from build123d import *

# Parameters (mm, degrees)
BOSS_EXTRUDE1_DEPTH            = 4.8
BOSS_EXTRUDE3_DEPTH            = 4.8
M3_CLEARANCE_HOLE2_D           = 3.4
M3_CLEARANCE_HOLE2_CSINK_D     = 3.45
M3_CLEARANCE_HOLE2_CSINK_ANGLE = 90
BOSS_EXTRUDE4_DEPTH            = 4.8
SKETCH11_W                     = 23
SKETCH11_H                     = 12.75
CUT_EXTRUDE1_DEPTH             = 4.8
M2_CLEARANCE_HOLE1_D           = 2.4
M2_CLEARANCE_HOLE1_CSINK_D     = 2.45
M2_CLEARANCE_HOLE1_CSINK_ANGLE = 90
CUT_EXTRUDE2_DEPTH             = 4.8
SKETCH16_W                     = 4.8
SKETCH16_H                     = 7
BOSS_EXTRUDE6_DEPTH            = 11
SKETCH17_R                     = 1.225
CUT_EXTRUDE3_DEPTH             = 11
CUT_EXTRUDE4_DEPTH             = 1.75


with BuildPart() as part:
    # Sketch1 → Boss-Extrude1 (new body)
    with BuildSketch(Plane(origin=(0, 0, 0), x_dir=(1, 0, 0), z_dir=(0, 1, 0))):
        with BuildLine():
            Line((6.83, 0), (-6.83, 0))
            ThreePointArc((-6.83, 0), (-8.951320344, -0.878679656), (-9.83, -3))
            Line((-9.83, -3), (-9.83, -7.63))
            ThreePointArc((-9.83, -7.63), (-10.708679656, -9.751320344), (-12.83, -10.63))
            Line((-12.83, -10.63), (-12.83, -16.63))
            Line((-12.83, -16.63), (12.83, -16.63))
            Line((12.83, -16.63), (12.83, -10.63))
            ThreePointArc((12.83, -10.63), (10.708679656, -9.751320344), (9.83, -7.63))
            Line((9.83, -7.63), (9.83, -3))
            ThreePointArc((9.83, -3), (8.951320344, -0.878679656), (6.83, 0))
        make_face()
    extrude(amount=BOSS_EXTRUDE1_DEPTH)

    # Sketch9 → Boss-Extrude3 (add)
    with BuildSketch(Plane(origin=(0, 4.8, 0), x_dir=(1, 0, 0), z_dir=(0, 1, 0))):
        with BuildLine():
            Line((12.83, -16.63), (12.83, -10.63))
            Line((12.83, -10.63), (20.51, -10.63))
            ThreePointArc((20.51, -10.63), (22.631320344, -9.751320344), (23.51, -7.63))
            Line((23.51, -7.63), (23.51, -5.44))
            ThreePointArc((23.51, -5.44), (24.388679656, -3.318679656), (26.51, -2.44))
            Line((26.51, -2.44), (27.36, -2.44))
            ThreePointArc((27.36, -2.44), (29.481320344, -1.561320344), (30.36, 0.56))
            Line((30.36, 0.56), (30.36, 6.56))
            Line((30.36, 6.56), (36.36, 6.56))
            Line((36.36, 6.56), (36.36, -16.63))
            Line((36.36, -16.63), (12.83, -16.63))
        make_face()
    extrude(amount=-BOSS_EXTRUDE3_DEPTH)

    # M3 Clearance Hole2 (through all)
    with Locations(Plane(origin=(0, 4.8, 0), x_dir=(1, 0, 0), z_dir=(0, 1, 0))):
        with Locations((0, -4.05), (30.821320344, -9.051320344)):
            CounterSinkHole(M3_CLEARANCE_HOLE2_D / 2, M3_CLEARANCE_HOLE2_CSINK_D / 2, counter_sink_angle=M3_CLEARANCE_HOLE2_CSINK_ANGLE)

    # Sketch10 → Boss-Extrude4 (add)
    with BuildSketch(Plane(origin=(0, 4.8, 0), x_dir=(1, 0, 0), z_dir=(0, 1, 0))):
        Polygon((-12.83, -16.63), (-12.83, -41.63), (77.88, -41.63), (77.88, 6.56), (36.36, 6.56), (36.36, -16.63), align=None)
    extrude(amount=-BOSS_EXTRUDE4_DEPTH)

    # Sketch11 → Cut-Extrude1 (cut)
    with BuildSketch(Plane(origin=(0, 4.8, 0), x_dir=(1, 0, 0), z_dir=(0, 1, 0))):
        with Locations((38.94, -30.255)):
            Rectangle(SKETCH11_W, SKETCH11_H)
    extrude(amount=-CUT_EXTRUDE1_DEPTH, mode=Mode.SUBTRACT)

    # M2 Clearance Hole1 (through all)
    with Locations(Plane(origin=(0, 4.8, 0), x_dir=(1, 0, 0), z_dir=(0, 1, 0))):
        with Locations((25.04, -30.255), (52.84, -30.255)):
            CounterSinkHole(M2_CLEARANCE_HOLE1_D / 2, M2_CLEARANCE_HOLE1_CSINK_D / 2, counter_sink_angle=M2_CLEARANCE_HOLE1_CSINK_ANGLE)

    # Sketch14 → Cut-Extrude2 (cut)
    with BuildSketch(Plane(origin=(0, 4.8, 0), x_dir=(1, 0, 0), z_dir=(0, 1, 0))):
        Polygon((-12.83, -16.59), (8.952290106, -41.63), (-12.83, -41.63), align=None)
        Polygon((36.36, 6.56), (77.88, -41.63), (77.88, 6.56), align=None)
    extrude(amount=-CUT_EXTRUDE2_DEPTH, mode=Mode.SUBTRACT)

    # Chamfer2
    # the kernel refuses this chamfer: 2, 1.418117079 mm, written as the material it takes off along each edge
    with BuildSketch(Plane(origin=(75.517763148, 3.466666667, 40.45827363), x_dir=(-0.07414602746519786, 0, 0.9972473948881141), z_dir=(0.5424620475376688, 0.83911156735298, 0.040332425115101794))) as chamfer2_piece_1:
        Polygon((-0.420862971, 1.22558177), (1.098498339, 1.22558177), (-0.677635367, -2.451163541), align=None)
    extrude(amount=2.692247612, mode=Mode.SUBTRACT)
    with BuildSketch(Plane(origin=(75.517763148, 1.333333333, 40.45827363), x_dir=(-0.07414602746519786, 0, 0.9972473948881141), z_dir=(0.5424620475376688, -0.83911156735298, 0.040332425115102044))) as chamfer2_piece_2:
        Polygon((-0.420862971, -1.22558177), (1.098498339, -1.22558177), (-0.677635367, 2.451163541), align=None)
    extrude(amount=2.692247612, mode=Mode.SUBTRACT)
    with BuildSketch(Plane(origin=(3.80892413, 4.8, 41.63), x_dir=(0, 0.02749587661058651, -0.9996219169112968), z_dir=(1, 0, 0))) as chamfer2_piece_3:
        with BuildLine():
            Line((2.05734639, 0), (-0.11309431, -2.054235587))
            Line((-0.11309431, -2.054235587), (-0.153079186, -2.053135752))
            ThreePointArc((-0.153079186, -2.053135752), (-0.068258454, -1.026795659), (-0.039984877, 0.001099835))
            Line((-0.039984877, 0.001099835), (0.001099835, 0.039984877))
            ThreePointArc((0.001099835, 0.039984877), (1.028995329, 0.011711299), (2.058446225, 0.039984877))
            Line((2.058446225, 0.039984877), (2.05734639, 0))
        make_face()
    extrude(amount=79.214441846, mode=Mode.SUBTRACT)
    with BuildSketch(Plane(origin=(-16.205706468, 4.8, 12.709430531), x_dir=(0.7541952701172161, 0.027495876610586487, -0.6560742879447683), z_dir=(0.6563224323571792, 0, 0.754480526445021))) as chamfer2_piece_4:
        with BuildLine():
            Line((2.05734639, 0), (-0.11309431, -2.054235587))
            Line((-0.11309431, -2.054235587), (-0.153079186, -2.053135752))
            ThreePointArc((-0.153079186, -2.053135752), (-0.068258454, -1.026795659), (-0.039984877, 0.001099835))
            Line((-0.039984877, 0.001099835), (0.001099835, 0.039984877))
            ThreePointArc((0.001099835, 0.039984877), (1.028995329, 0.011711299), (2.058446225, 0.039984877))
            Line((2.058446225, 0.039984877), (2.05734639, 0))
        make_face()
    extrude(amount=43.475129959, mode=Mode.SUBTRACT)
    with BuildSketch(Plane(origin=(-16.205706468, 0, 12.709430531), x_dir=(0.7541952701172161, -0.02749587661058636, -0.6560742879447683), z_dir=(0.6563224323571792, 0, 0.754480526445021))) as chamfer2_piece_5:
        with BuildLine():
            Line((2.05734639, 0), (-0.11309431, 2.054235587))
            Line((-0.11309431, 2.054235587), (-0.153079186, 2.053135752))
            ThreePointArc((-0.153079186, 2.053135752), (-0.068258454, 1.026795659), (-0.039984877, -0.001099835))
            Line((-0.039984877, -0.001099835), (0.001099835, -0.039984877))
            ThreePointArc((0.001099835, -0.039984877), (1.028995329, -0.011711299), (2.058446225, -0.039984877))
            Line((2.058446225, -0.039984877), (2.05734639, 0))
        make_face()
    extrude(amount=43.475129959, mode=Mode.SUBTRACT)
    with BuildSketch(Plane(origin=(33.002764366, 4.8, -10.456560337), x_dir=(-0.7573031224660502, 0.027495876610586473, 0.6524844499852744), z_dir=(0.6527312366273116, 0, 0.757589554264696))) as chamfer2_piece_6:
        with BuildLine():
            Line((2.05734639, 0), (-0.11309431, 2.054235587))
            Line((-0.11309431, 2.054235587), (-0.153079186, 2.053135752))
            ThreePointArc((-0.153079186, 2.053135752), (-0.068258454, 1.026795659), (-0.039984877, -0.001099835))
            Line((-0.039984877, -0.001099835), (0.001099835, -0.039984877))
            ThreePointArc((0.001099835, -0.039984877), (1.028995329, -0.011711299), (2.058446225, -0.039984877))
            Line((2.058446225, -0.039984877), (2.05734639, 0))
        make_face()
    extrude(amount=73.896373517, mode=Mode.SUBTRACT)
    with BuildSketch(Plane(origin=(33.002764366, 0, -10.456560337), x_dir=(-0.7573031224660502, -0.02749587661058634, 0.6524844499852744), z_dir=(0.6527312366273116, 0, 0.757589554264696))) as chamfer2_piece_7:
        with BuildLine():
            Line((2.05734639, 0), (-0.11309431, -2.054235587))
            Line((-0.11309431, -2.054235587), (-0.153079186, -2.053135752))
            ThreePointArc((-0.153079186, -2.053135752), (-0.068258454, -1.026795659), (-0.039984877, 0.001099835))
            Line((-0.039984877, 0.001099835), (0.001099835, 0.039984877))
            ThreePointArc((0.001099835, 0.039984877), (1.028995329, 0.011711299), (2.058446225, 0.039984877))
            Line((2.058446225, 0.039984877), (2.05734639, 0))
        make_face()
    extrude(amount=73.896373517, mode=Mode.SUBTRACT)
    with BuildSketch(Plane(origin=(77.88, 9.943365976, 41.63), x_dir=(-0.6316538610797438, 0, -0.7752505400082296), z_dir=(0, -1, 0))) as chamfer2_piece_8:
        with BuildLine():
            Line((2.05734639, 0), (0.837656572, -1.154387784))
            Line((0.837656572, -1.154387784), (0.80664655, -1.179653939))
            ThreePointArc((0.80664655, -1.179653939), (0.418742927, -0.57726344), (-0.031010022, -0.025266154))
            Line((-0.031010022, -0.025266154), (0.001099835, 0.039984877))
            ThreePointArc((0.001099835, 0.039984877), (1.028995329, 0.011711299), (2.058446225, 0.039984877))
            Line((2.058446225, 0.039984877), (2.05734639, 0))
        make_face()
    extrude(amount=15.086731952, mode=Mode.SUBTRACT)
    with BuildSketch(Plane(origin=(3.80892413, 0, 41.63), x_dir=(0, -0.02749587661058639, -0.9996219169112968), z_dir=(1, 0, 0))) as chamfer2_piece_9:
        with BuildLine():
            Line((2.05734639, 0), (-0.11309431, 2.054235587))
            Line((-0.11309431, 2.054235587), (-0.153079186, 2.053135752))
            ThreePointArc((-0.153079186, 2.053135752), (-0.068258454, 1.026795659), (-0.039984877, -0.001099835))
            Line((-0.039984877, -0.001099835), (0.001099835, -0.039984877))
            ThreePointArc((0.001099835, -0.039984877), (1.028995329, -0.011711299), (2.058446225, -0.039984877))
            Line((2.058446225, -0.039984877), (2.05734639, 0))
        make_face()
    extrude(amount=79.214441846, mode=Mode.SUBTRACT)

    # Sketch16 → Boss-Extrude6 (add)
    with BuildSketch(Plane.XZ):
        with Locations((25.04, 30.255)):
            Rectangle(SKETCH16_W, SKETCH16_H)
        with Locations((52.84, 30.255)):
            Rectangle(SKETCH16_W, SKETCH16_H)
    extrude(amount=BOSS_EXTRUDE6_DEPTH)

    # Sketch17 → Cut-Extrude3 (cut)
    with BuildSketch(Plane.XZ.offset(11)):
        with Locations(Location((25.04, 30.255, 0), (0, 0, 270))):
            Circle(SKETCH17_R)
        with Locations(Location((52.84, 30.255, 0), (0, 0, 270))):
            Circle(SKETCH17_R)
    extrude(amount=-CUT_EXTRUDE3_DEPTH, mode=Mode.SUBTRACT)

    # Sketch18 → Cut-Extrude4 (cut)
    with BuildSketch(Plane.XZ.offset(11)):
        Polygon((25.04, 27.945598923), (27.04, 29.100299462), (27.04, 31.409700538), (25.04, 32.564401077), (23.04, 31.409700538), (23.04, 29.100299462), align=None)
        Polygon((52.84, 27.945598923), (54.84, 29.100299462), (54.84, 31.409700538), (52.84, 32.564401077), (50.84, 31.409700538), (50.84, 29.100299462), align=None)
    extrude(amount=-CUT_EXTRUDE4_DEPTH, mode=Mode.SUBTRACT)


solid = part.part
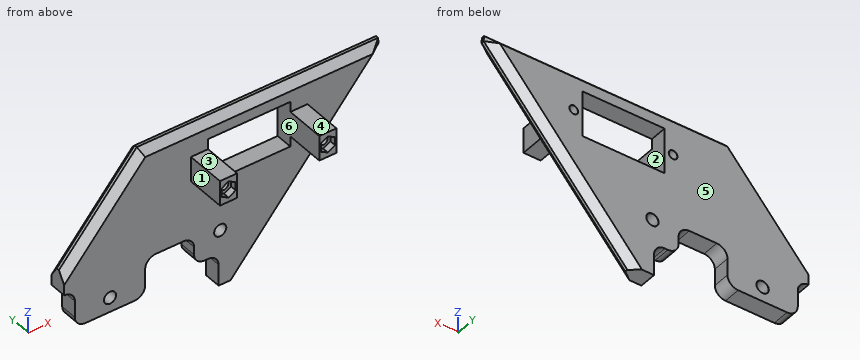
CAD build for the part. Positions are in the model's coordinates, mm. Face numbers are marked on the shaded views. A direction names the side the tool comes from. Coordinates: 2 decimals unless noted, no trailing zeros. Write each loop counter-clockwise with the first axis right and the second up, starting at its lowest first coordinate (ties: lowest second). Pieces come first, ordered by that corner, then holes. Notation, with made-up numbers: M 9.25,51.5 L 57.25,51.5 A26 ccw 57.25,67.5 Z; hole C 74.5,0 d7. An arc over 180 degrees is marked long. Answer as a JSON object with one key per item and string values. Group by question number.
1) Saw through at C-C (x = 0). Write the cut outline in (y, z) (3 decimals).
2) Mould opens along Z. For the marked faces 1, 2 and 3 say: +Z half, -Z half, draft (parallel to the pull), parting line (faces both ways), or undercut.
3) Saw through at A-A (y = -3.25). Write the cut outline in (x, z) (3 decimals).
4) Wall check: line 1 (Z direction, x = 30, y = 0.25); line 2 (Y direction, x = 35.5, z = 16); line 3 (Z direction, x = 32, y = 0.5). Give the ranges that are in metal, low to high. Write a range as from..to.
5) Saw through at D-D (z = 25). Write the cut outline in (x, y).
6) Pin check, flat tips, straight feed: pin 1 Ø0.9 at (x, y) = (27, 3.5) entering from -Z; pin 2 Ø1.4 at (y, z) = (-9.5, 30.5) entering from -X; pin 3 Ø2.5 at (x, y) = (53, -8) entering from +Z (3 decimals); pin 4 Ø4.5 at (x, z) = (53.5, 30.5) entering from -Y. Stop position of each tip, or through.
7) Tool access for the marked faces 4, 5 and 6: list every direction of +Z, -Z, +X, -X, +Y, -Y with a clear straight run to the whole face (end or side of a thin tool).
8) Saw through at B-B (z = 4.05). Write the cut outline in (x, y) (3 decimals), plus the area to 3 significant figures.
Values follow:
{
 "1": {"outline": "M 0,0 L 4.8,0 L 4.8,2.325 L 4.775,2.35 L 0,2.35 Z; M 0,5.75 L 4.775,5.75 L 4.8,5.775 L 4.8,28.292 L 2.8,31.339 L 2,31.339 L 0,28.292 Z"},
 "2": {"face 1": "draft", "face 2": "undercut", "face 3": "+Z half"},
 "3": {"outline": "M 22.64,26.755 L 27.44,26.755 L 27.44,33.755 L 22.64,33.755 Z; M 50.44,26.755 L 55.24,26.755 L 55.24,33.755 L 50.44,33.755 Z; hole C 25.04,30.255 d2.45; hole C 52.84,30.255 d2.45"},
 "4": {"line 1": "z = 0.86..7.56, 10.54..23.88, 36.63..39.88", "line 2": "y = 0..4.8", "line 3": "z = -6.56..7.83, 10.28..23.88, 36.63..40.13"},
 "5": {"outline": "M -5.51,2 L -2.86,0 L 27.44,0 L 27.44,4.8 L -2.86,4.8 L -5.51,2.8 Z; M 50.44,0 L 60.91,0 L 63.55,2 L 63.55,2.8 L 60.91,4.8 L 50.44,4.8 Z"},
 "6": {"pin 1": "stops at z = 2.44", "pin 2": "stops at x = 22.64", "pin 3": "stops at z = 33.755", "pin 4": "stops at y = -11"},
 "7": {"face 4": "+Z, +X, -X, -Y", "face 5": "+Z, -Z, +X, -X, +Y", "face 6": "+Y, -Y"},
 "8": {"outline": "M -9.83,0 L -1.7,0 L -1.7,4.775 L -1.725,4.8 L -9.83,4.8 Z; M 1.7,0 L 9.83,0 L 9.83,4.8 L 1.725,4.8 L 1.7,4.775 Z; M 23.851,0 L 42.862,0 L 45.501,2 L 45.501,2.8 L 42.862,4.8 L 23.851,4.8 Z", "area": "177 mm2"}
}
